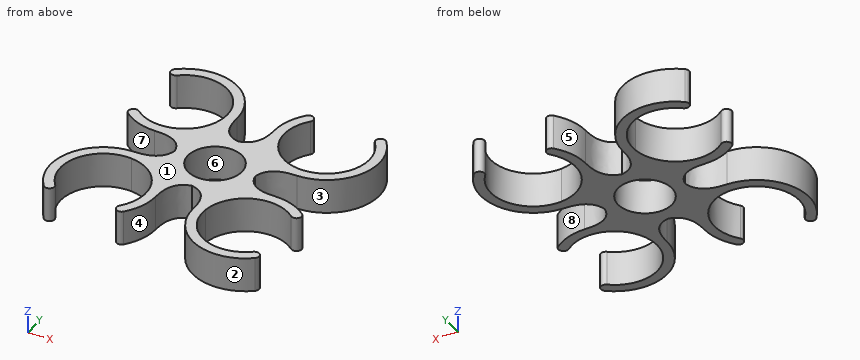
from build123d import *

# Parameters (mm, degrees)
ESQUISSE2_R        = 13.315895319
BOSS_EXTRU_1_DEPTH = 17


with BuildPart() as part:
    # Esquisse2 → Boss.-Extru.1 (new body)
    with BuildSketch(Plane.XY):
        with BuildLine():
            ThreePointArc((-41.970273906, 58.288916899), (-45.477336755, 58.674660716), (-45.106104784, 62.183289358))
            ThreePointArc((-45.106104784, 62.183289358), (-17.574909645, 65.492333679), (-2.716007813, 42.080167687))
            add(Edge.make_bspline(
                [(-2.716007813, 42.080167687), (-3.035124512, 28.491732954), (6.642053999, 26.657753906)],
                knots=[0, 0, 0, 1, 1, 1], degree=2))
            add(Edge.make_bspline(
                [(16, 42.080237959), (16.319218738, 28.491805623), (6.642053999, 26.657753906)],
                knots=[0, 0, 0, 1, 1, 1], degree=2))
            ThreePointArc((16, 42.080237959), (17.620066034, 51.034561919), (22.226418394, 58.882239885))
            ThreePointArc((22.226418394, 58.882239885), (25.715663474, 59.135975829), (26.044340034, 55.652990776))
            ThreePointArc((26.044340034, 55.652990776), (22.521938117, 34.151609621), (39.967073041, 21.098488371))
            ThreePointArc((39.967073041, 21.098488371), (60.505936251, 32.073055278), (58.288905312, 55.254314833))
            ThreePointArc((58.288905312, 55.254314833), (58.674649129, 58.761377683), (62.18327777, 58.390145711))
            ThreePointArc((62.18327777, 58.390145711), (65.492322092, 30.858950572), (42.080156099, 16.000048741))
            add(Edge.make_bspline(
                [(42.080156099, 16.000048741), (28.491721366, 16.319165439), (26.657742318, 6.641986928)],
                knots=[0, 0, 0, 1, 1, 1], degree=2))
            add(Edge.make_bspline(
                [(42.080226372, -2.715959073), (28.491794035, -3.035177811), (26.657742318, 6.641986928)],
                knots=[0, 0, 0, 1, 1, 1], degree=2))
            ThreePointArc((42.080226372, -2.715959073), (51.034550331, -4.336025106), (58.882228297, -8.942377467))
            ThreePointArc((58.882228297, -8.942377467), (59.135964241, -12.431622547), (55.652979189, -12.760299107))
            ThreePointArc((55.652979189, -12.760299107), (34.151598033, -9.23789719), (21.098476784, -26.683032113))
            ThreePointArc((21.098476784, -26.683032113), (32.07304369, -47.221895323), (55.254303246, -45.004864384))
            ThreePointArc((55.254303246, -45.004864384), (58.761366095, -45.390608201), (58.390134124, -48.899236843))
            ThreePointArc((58.390134124, -48.899236843), (30.858938985, -52.208281164), (16.000037153, -28.796115172))
            add(Edge.make_bspline(
                [(16.000037153, -28.796115172), (16.319153851, -15.207680439), (6.64197534, -13.373701391)],
                knots=[0, 0, 0, 1, 1, 1], degree=2))
            add(Edge.make_bspline(
                [(-2.71597066, -28.796185444), (-3.035189399, -15.207753108), (6.64197534, -13.373701391)],
                knots=[0, 0, 0, 1, 1, 1], degree=2))
            ThreePointArc((-2.71597066, -28.796185444), (-4.336036694, -37.750509404), (-8.942389054, -45.59818737))
            ThreePointArc((-8.942389054, -45.59818737), (-12.431634134, -45.851923314), (-12.760310694, -42.368938261))
            ThreePointArc((-12.760310694, -42.368938261), (-9.237908778, -20.867557106), (-26.683043701, -7.814435856))
            ThreePointArc((-26.683043701, -7.814435856), (-47.221906911, -18.789002763), (-45.004875972, -41.970262318))
            ThreePointArc((-45.004875972, -41.970262318), (-45.390619789, -45.477325168), (-48.899248431, -45.106093196))
            ThreePointArc((-48.899248431, -45.106093196), (-52.208292752, -17.574898057), (-28.79612676, -2.715996226))
            add(Edge.make_bspline(
                [(-28.79612676, -2.715996226), (-15.207692026, -3.035112924), (-13.373712979, 6.642065587)],
                knots=[0, 0, 0, 1, 1, 1], degree=2))
            add(Edge.make_bspline(
                [(-28.796197032, 16.000011588), (-15.207764695, 16.319230326), (-13.373712979, 6.642065587)],
                knots=[0, 0, 0, 1, 1, 1], degree=2))
            ThreePointArc((-28.796197032, 16.000011588), (-37.750520991, 17.620077621), (-45.598198957, 22.226429982))
            ThreePointArc((-45.598198957, 22.226429982), (-45.851934901, 25.715675062), (-42.368949849, 26.044351622))
            ThreePointArc((-42.368949849, 26.044351622), (-20.867568694, 22.521949705), (-7.814447444, 39.967084628))
            ThreePointArc((-7.814447444, 39.967084628), (-18.789014351, 60.505947838), (-41.970273906, 58.288916899))
        make_face()
        with Locations((6.64201467, 6.642026257)):
            Circle(ESQUISSE2_R, mode=Mode.SUBTRACT)
    extrude(amount=BOSS_EXTRU_1_DEPTH)


solid = part.part
Could you check a few things on this model? Use its own coordinates, in mm. Face numbers are marked on the shaded views. A direction names the side the tool comes from. Coordinates: 2 decimals unless noted, no trailing zeros. Order: outer loops, then holes, each group sorted by start corner. A loop starts at its lowest first (then second) coordinate and runs counter-clockwise, first axis right, second up.
Q1. Will these pins go through, and if not, where does the flat tip stop? pin 1 (8 mm diameter, centred on y = 23.5, z = 6.5, fed in from +X); pin 2 (5 mm diameter, centred on y = 45.5, z = 4, fed in from +X); pin 3 (3 mm diameter, centred on y = 44.5, z = 8, fed in from -X).
Q2. Which directions (+Z, -Z, +X, -X, +Y, -Y) give clear straight access to the entire face, cutting with the end or side of a thin tool? Please do the marked faces 4, 5, 6, 7 and 8.
Q3. Suppose I cut it at B-B on x = 29. Give the number of separate pieces and of enclosed holes in the cut face, and give its area (3 significant figures).
Q4. Thinking about a two-plate mould opening in X: for the marked faces 1, 2 and 3, which applies, released by +X, released by -X, zero draft, split by the parting line, or undercut?
Q5. Please list where these lines run through material, in increasing order: L1, parallel to Y at x = -39.5, z = 3.25; L2, parallel to Y at x = -34, z = 5; L3, parallel to X at y = 42, z = 8.
Q6. Suppose I cut it at A-A on y = -35.5. Please give me the cut outline in (x, z), and give its area (3 significant figures).
Answer:
1. pin 1: stops at x = 63.58
1. pin 2: stops at x = 67.98
1. pin 3: stops at x = -8.1
2. face 4: +Z, -Z, -Y
2. face 5: +Z, -Z, +Y
2. face 6: +Z, -Z
2. face 7: +Z, -Z, -X
2. face 8: +Z, -Z, +X
3. separate pieces: 3
3. enclosed holes: 0
3. area: 569 mm2
4. face 1: zero draft
4. face 2: undercut
4. face 3: released by +X
5. L1: y = -10.7 to -5.06, 18.34 to 23.98, 60.02 to 65.66
5. L2: y = -8.39 to -3.26, 16.54 to 21.68, 62.32 to 67.46
5. L3: x = -7.72 to -2.72, 16 to 21, 63 to 68
6. outline: (-53.82, 0) - (-48.59, 0) - (-48.59, 17) - (-53.82, 17) - close; (-8.84, 0) - (-3.62, 0) - (-3.62, 17) - (-8.84, 17) - close; (16.9, 0) - (22.13, 0) - (22.13, 17) - (16.9, 17) - close
6. area: 266 mm2
